Geometry: final body of the model. Coordinates: model frame, mm. A direction names the side the tool comes from. Give positions to 0.01 mm unless a question says otherwise; leave off trailing zeros. Write each loop counter-clockwise with the first axis right and the second up, starting at its lowest first coordinate (ties: lowest second). Pieces come first, ordered by that corner, then holes. Notation, with made-up numbers: (-7.75, 54.5) -> (30.25, 54.5) arc R25 cw to (30.25, 75.5) -> close; hole circle Ø7 at (88, 48). An arc over 180 degrees is marked (long way). Use CSV: the item, a comma, the result in double quotes. Start each with the question number.
1) Section B-B (x = 0.65). Output: boundary loops of the cut face in (y, z), plus the area to 3 significant figures.
2) Draft query along Y for faces 3 (the face through (1, -25, 9)), 4 (the face through (1, 0, 20)), 5 (the face through (0.81, 24.57, 19.55)), 6 (the face through (0.789, -18.567, -9.086)). Return one class per face: pulls with the +Y half, pulls with the -Y half, needs draft (parallel to the pull), parting line crosses it, or undercut.
3) Section A-A (y = 20). Output: boundary loops of the cut face in (x, z), plus the area to 3 significant figures.
4) Section C-C (z = 15). Output: boundary loops of the cut face in (x, y), plus the area to 3 significant figures.
5) Section D-D (z = -10). Output: boundary loops of the cut face in (x, y).
6) Material intervals for line 1 (Y direction, x = 0.95, z = -10); line 2 (Y direction, x = 0.75, z = 15); line 3 (Y direction, x = 0.2, z = 7), sorted ascending. Write a range as [from, to].
7) Contact query for a flat-ended pin moving along its axis: P1, Ø1.5, axis at y = -30.5, z = -1.5, coming from the +X side. Output: stop coordinate, or through.
8) Set-up query: faces 1 (the face through (1, -35, -2)), 2 (the face through (1, 25, 0)). Return all of +Z, -Z, +X, -X, +Y, -Y with unobstructed straight access to the full face (end or side cutting, diameter ignored); none if empty.
```python
from build123d import *

# Parameters (mm, degrees)
BOSS_EXTRUDE1_DEPTH      = 1.6002
M3_CLEARANCE_HOLE1_D     = 3.4
M3_CLEARANCE_HOLE1_DEPTH = 6
M3_CLEARANCE_HOLE1_TIP   = 1.021463052
FILLET1_R                = 1.5


with BuildPart() as part:
    # Sketch1 → Boss-Extrude1 (new body)
    with BuildSketch(Plane(origin=(0, 0, 0), x_dir=(0, 0, -1), z_dir=(1, 0, 0))):
        Polygon((-20, 25), (20, 25), (20, -25), (20, -45), (2, -45), (2, -25), (-20, -25), align=None)
    extrude(amount=BOSS_EXTRUDE1_DEPTH)

    # M3 Clearance Hole1
    with Locations(Plane(origin=(1.6002, 0, 0), x_dir=(0, 0, -1), z_dir=(1, 0, 0))):
        with Locations((10, 20), (10, -20), (-15, 0)):
            Hole(M3_CLEARANCE_HOLE1_D / 2, depth=M3_CLEARANCE_HOLE1_DEPTH)
            with Locations((0, 0, -(M3_CLEARANCE_HOLE1_DEPTH + M3_CLEARANCE_HOLE1_TIP / 2))):  # 118° drill point
                Cone(0, M3_CLEARANCE_HOLE1_D / 2, M3_CLEARANCE_HOLE1_TIP, mode=Mode.SUBTRACT)

    # Fillet1
    fillet1_edges = [part.edges().sort_by_distance(p)[0] for p in [
        (0.8001, -45, -20),
        (0.8001, -45, -2),
        (0.8001, -25, -2),
        (0.8001, -25, 20),
        (0.8001, 25, 20),
        (0.8001, 25, -20),
    ]]
    fillet(fillet1_edges, radius=FILLET1_R)


solid = part.part
```
Answers follow:
1,outline,"(-45, -18.5) arc R1.5 ccw to (-43.5, -20) -> (23.5, -20) arc R1.5 ccw to (25, -18.5) -> (25, 18.5) arc R1.5 ccw to (23.5, 20) -> (-23.5, 20) arc R1.5 ccw to (-25, 18.5) -> (-25, -0.5) arc R1.5 cw to (-26.5, -2) -> (-43.5, -2) arc R1.5 ccw to (-45, -3.5) -> close; hole circle Ø3.4 at (-20, -10); hole circle Ø3.4 at (0, 15); hole circle Ø3.4 at (20, -10)"
1,area,"2,330 mm^2"
2,face 3,"pulls with the -Y half"
2,face 4,"needs draft"
2,face 5,"pulls with the +Y half"
2,face 6,"undercut"
3,outline,"(0, -20) -> (1.6, -20) -> (1.6, -11.7) -> (0, -11.7) -> close; (0, -8.3) -> (1.6, -8.3) -> (1.6, 20) -> (0, 20) -> close"
3,area,"58.6 mm^2"
4,outline,"(0, -25) -> (1.6, -25) -> (1.6, -1.7) -> (0, -1.7) -> close; (0, 1.7) -> (1.6, 1.7) -> (1.6, 25) -> (0, 25) -> close"
4,area,"74.6 mm^2"
5,outline,"(0, -45) -> (1.6, -45) -> (1.6, -21.7) -> (0, -21.7) -> close; (0, -18.3) -> (1.6, -18.3) -> (1.6, 18.3) -> (0, 18.3) -> close; (0, 21.7) -> (1.6, 21.7) -> (1.6, 25) -> (0, 25) -> close"
6,line 1,"y = [-45, -21.7], [-18.3, 18.3], [21.7, 25]"
6,line 2,"y = [-25, -1.7], [1.7, 25]"
6,line 3,"y = [-25, 25]"
7,P1,"stops at x = 1.6"
8,face 1,"+Z, +X, -X, -Y"
8,face 2,"+Z, -Z, +X, -X, +Y"
